Could you check a few things on this model? Use its own coordinates, in mm. Coordinates: 2 decimals unless noted, no trailing zeros. Answer as CSV lines item,"result". Start each with the question number.
Item 1: If I drill on line 1 along X through (y, z) = (0.3, -298); line 2 along X through (y, z) = (-0.1, -217), over which ranges is the centre line in solid material (lowest first)? Write a range as [from, to].
Item 2: We'd pull the mould along X, two halves only. Please class faces 1 (the cylindrical face through (0.209, 0.014, -204.783)), 2 (the flat face through (-8, 0.992, -294)): +X half, -X half, draft (parallel to the pull), parting line (faces both ways), or undercut.
Item 3: I'm going to push a flat-ended pin straight in: P1, Ø5.5, axis at x = 0, z = -371.475, coming from the +Y side. Where does the tip first touch, or does it pass through?
Item 4: Suppose I cut it at A-A, the plane y = 0.6. State how many separate pieces and enclosed holes the cut face has, and give its area (3 significant figures).
```python
from build123d import *

# Parameters (mm, degrees)
BOSS_EXTRUDE1_DEPTH      = 0.99187
BOSS_EXTRUDE1_DEPTH_BACK = 0.99187
SKETCH3_W                = 34.925
SKETCH3_H                = 914.4
CUT_EXTRUDE1_REACH       = 459.538
SKETCH4_R                = 4.7625
LPATTERN1_COUNT          = 53
LPATTERN1_PITCH          = 19.05
SKETCH5_W                = 34.925
SKETCH5_H                = 1.98374
CUT_EXTRUDE2_DEPTH       = 584.2


with BuildPart() as part:
    # Sketch3 → Boss-Extrude1 (new, two sides: drawn at the far end of the back side and taken through both)
    with BuildSketch(Plane(origin=(0, 0, 0), x_dir=(1, 0, 0), z_dir=(0, 1, 0)).offset(-BOSS_EXTRUDE1_DEPTH_BACK)):
        Rectangle(SKETCH3_W, SKETCH3_H)
    extrude(amount=BOSS_EXTRUDE1_DEPTH + BOSS_EXTRUDE1_DEPTH_BACK)

    # Sketch4 → Cut-Extrude1 (cut, up to next)
    with BuildSketch(Plane(origin=(0, 0.99187, 0), x_dir=(1, 0, 0), z_dir=(0, 1, 0)), mode=Mode.PRIVATE) as cut_extrude1_sk1:
        with Locations(Location((0, -447.675, 0), (0, 0, 270))):
            Circle(SKETCH4_R)
    cut_extrude1_tool1 = extrude(cut_extrude1_sk1.sketch, amount=-CUT_EXTRUDE1_REACH, mode=Mode.PRIVATE) & part.part
    cut_extrude1 = cut_extrude1_tool1.solids().sort_by_distance((0, 0.99187, 447.675))[0]
    add(cut_extrude1, mode=Mode.SUBTRACT)

    # LPattern1: Cut-Extrude1 ×53
    with Locations(*[(0, 0, -i * LPATTERN1_PITCH) for i in range(1, LPATTERN1_COUNT)]):
        add(cut_extrude1, mode=Mode.SUBTRACT)

    # Sketch5 → Cut-Extrude2 (cut)
    with BuildSketch(Plane.XY.offset(457.2)):
        Rectangle(SKETCH5_W, SKETCH5_H)
    extrude(amount=-CUT_EXTRUDE2_DEPTH, mode=Mode.SUBTRACT)


solid = part.part
```
Ans:
1,line 1,"x = [-17.46, -3.91], [3.91, 17.46]"
1,line 2,"x = [-17.46, -4.29], [4.29, 17.46]"
2,face 1,"undercut"
2,face 2,"draft"
3,P1,"passes through"
4,separate pieces,"1"
4,enclosed holes,"17"
4,area,"10,300 mm^2"
